The listing builds one solid part. Answer for the finished solid, in the listing's coordinates (mm). A direction names the side the tool comes from. Give positions to 0.01 mm unless a question says otherwise; leave off trailing zeros. Write each loop counter-clockwise with the first axis right and the second up, starting at its lowest first coordinate (ties: lowest second). Pieces come first, ordered by that corner, then holes. Notation, with made-up numbers: (-9.5, -37.5) - (47.5, -37.5) arc R14 cw to (47.5, -15.5) - close; hole circle Ø4 at (46, 35.25). An arc over 180 degrees is marked (long way). Answer as CSV lines item,"result". Start each with the question number.
(1) Straight lines are drawn through the part: probe 1 along X at (y, z) = (-1, 1.5); probe 2 along Y at (x, z) = (-31, 7); probe 3 along X at (y, z) = (-22, 15). For each, find the intervals that lie inside material, in ascending order.
(2) Find section A-A (x = 12). Write down the section's boundary in (y, z), then the cut area to 3 significant figures.
(3) For faces 4 (the face through (39.07, -12.31, 7.87)), 5 (the face through (-11.2, 8.683, 7.874)), 6 (the face through (-19.366, -28.892, 8.381)), determine the directions among +Z, -Z, +X, -X, +Y, -Y from which every point of the face is accessible in a straight line to the end or side of a thin tool.
(4) Each of these flat-tipped pins is pushed along its axis until it touches: pin 1 Ø5 at (y, z) = (1.5, 10) entering from -X; pin 2 Ø2 at (y, z) = (8, 12) entering from +X; pin 3 Ø1.9 at (y, z) = (-39, 10.5) entering from +X. Where does it stop, or does it pass through?
(5) For a pull along Y with two mould halves and no side action, classify faces 1 (the face through (4.032, 26, 8)), 2 (the face through (16.282, -1.885, 8.381)), 3 (the face through (-12.273, -53.925, 7.874)) as pulls with the +Y half, pulls with the -Y half, needs draft (parallel to the pull), parting line crosses it, or undercut.
from build123d import *

# Parameters (mm, degrees)
F1_DEPTH = 17
F2_T     = 1


with BuildPart() as f1:
    # F0 (on Top) → F1 (new body)
    with BuildSketch(Plane.XY):
        Polygon((-27.7714431286, 3.3306172118), (-42.2787889838, 11.6773098707), (-46.0546761751, 6.3115782104), (-33.8464085439, -2.2794293716), (-43.471172452, -8.9906910434), (-36.515597254, -11.5741910413), (-25.3866743296, -5.4135369137), (-21.0145972669, -8.9906910434), (-30.7524055243, -15.5488057062), (-21.0145972669, -21.5107295662), (-27.3739825934, -24.6904212981), (-38.5029055178, -18.5297690332), (-44.0673679113, -22.703114897), (-31.9447889924, -30.2548836917), (-45.6572137773, -38.0053855479), (-43.173648768, -42.3993846747), (-29.0093820945, -34.3934938956), (-29.0093820945, -47.5444607437), (-22.2069825977, -44.1660396755), (-22.2069825977, -30.8510754257), (-16.4437890053, -26.8764607608), (-16.4437890053, -41.7812690139), (-5.3148670122, -35.2231524885), (-5.3148670122, -41.5825396776), (-18.0336348712, -50.1279607415), (-18.0336348712, -55.4936937988), (-4.3212124147, -49.1343066096), (-4.3212124147, -62.0518065989), (2.2369034123, -62.0518065989), (2.2369034123, -49.5317690074), (13.3658256382, -55.4936937988), (13.3658256382, -47.7431900799), (1.6407109797, -40.9863442183), (1.6407109797, -35.0244231522), (13.5645577684, -40.787614882), (13.5645577684, -28.2675754279), (18.5328256339, -30.6523460895), (20.3214026988, -45.3584231436), (26.6807861626, -48.7368442118), (26.6807861626, -35.2231524885), (39.9957485497, -42.5761900842), (43.2241563976, -36.7301531906), (28.4681427782, -28.5813113274), (41.9830568135, -21.908191964), (34.6300154924, -18.3310378343), (22.1099797636, -25.4853442311), (16.9429797679, -22.3056524992), (27.6744421571, -16.1449983716), (15.3531348333, -8.394498378), (23.1036357582, -5.6122676469), (35.2262109518, -13.5614983737), (41.1881357431, -9.7856139764), (28.4693632275, -1.4389213175), (43.1467061942, 5.2062330151), (38.8033650815, 12.0747713372), (25.2896733582, 3.5293472465), (25.2896733582, 17.0430392027), (18.7315568328, 13.6646172032), (18.7315568328, 0), (13.7632861733, -3.8236908149), (13.7632861733, 11.2798474729), (1.8394411309, 3.5293472465), (1.8394411309, 8.6963474751), (14.3594788387, 17.2417722642), (14.3594788387, 25.5884621292), (3.0318258796, 17.4405016005), (3.0318258796, 31.3516557217), (-5.3148670122, 31.3516557217), (-5.3148670122, 18.2354263961), (-16.2450578064, 24.1973474622), (-16.2450578064, 17.0430392027), (-4.3212124147, 10.8823850751), (-4.3212124147, 4.1255401447), (-16.2450578064, 10.0874630734), (-16.2450578064, -3.8236908149), (-23.2006367296, 0), (-23.2006367296, 13.2671557367), (-27.7714431286, 16.0493850708), align=None)
    extrude(amount=F1_DEPTH)

    # F2
    f2_openings = [f1.faces().sort_by_distance(p)[0] for p in [
        (-0.933502, -15.354262, 17),
    ]]
    offset(amount=F2_T, openings=f2_openings, kind=Kind.INTERSECTION)


solid = f1.part
Result set:
1,probe 1,"-37.4 to -35.66, -21.38 to -19.31, -17.25 to -16.25, 13.76 to 14.76, 15.79 to 17.43, 29.44 to 31.86"
1,probe 2,"-36.67 to -35.52, -22.68 to -21.54, -16.57 to -14.51, -9.66 to -8.52, 5.19 to 6.34"
1,probe 3,"-44.8 to -43.13, -32.23 to -30.17, -24.23 to -21.99, 17.48 to 19.48, 26.19 to 28.21, 41.8 to 44.06"
2,outline,"(-55.9, -1) - (-45.8, -1) - (-45.8, 17) - (-46.96, 17) - (-46.96, 0) - (-54.76, 0) - (-54.76, 17) - (-55.9, 17) - close; (-41.14, -1) - (11.33, -1) - (11.33, 17) - (10.13, 17) - (10.13, 0) - (-40.03, 0) - (-40.03, 17) - (-41.14, 17) - close; (14.42, -1) - (25.12, -1) - (25.12, 17) - (23.89, 17) - (23.89, 0) - (15.63, 0) - (15.63, 17) - (14.42, 17) - close"
2,area,"193 mm^2"
3,face 4,"+Z, -Z, +X"
3,face 5,"+Z, -Z"
3,face 6,"+Z"
4,pin 1,"x = -44.51"
4,pin 2,"x = 43.2"
4,pin 3,"x = 43.64"
5,face 1,"needs draft"
5,face 2,"undercut"
5,face 3,"pulls with the -Y half"
